Geometry: final body of the model. Coordinates: model frame, mm. Face numbers are marked on the shaded views. A direction names the side the tool comes from. Give positions to 0.01 mm unless a question says otherwise; leave off trailing zeros. Write each loop counter-clockwise with the first axis right and the second up, starting at its lowest first coordinate (ties: lowest second). Pieces come first, ordered by that corner, then holes. Notation, with made-up numbers: M 64,69.5 L 81,69.5 A17 ccw 81,94.5 Z; hole C -34.5,46.5 d7. An arc over 180 degrees is marked long. Use a Markdown table: item, result. Add a question column.
(1) Cut plane D-D (x = -25.5). Output: boundary loops of the cut face in (y, z) (3 decimals).
(2) Draft query along Y for the marked faces 3, 4 and 5. Return one class per face: released by +Y, released by -Y, zero draft, split by the parting line, or undercut.
(3) Cut plane B-B (z = 6.5). Output: boundary loops of the cut face in (x, y) (1 decimal), plus the area to 3 significant figures.
(4) Material intervals for L1, parallel to Z at x = -52.5, y = 12.7 (3 decimals); L2, parallel to Z at x = -32.5, y = 12.7; L3, parallel to X at y = 13, z = 7.25, sorted ascending.
(5) Pin query (flat end, axial travel): pin 1 Ø3 at (x, z) = (-33.5, -10) entering from +Y; pin 2 Ø2 at (y, z) = (14.5, 4.5) entering from -X; pin 3 Ø6 at (y, z) = (8, 4) entering from -X. Return the tip coordinate at first contact, or that it passes through.
(6) Reachability of the marked faces 1 and 2 from +Z, -Z, +X, -X, +Y, -Y: full face, straight path, thin tool, end or side. Return the list, or none.
(7) Cut plane A-A (y = 12.7). Output: boundary loops of the cut face in (x, z) (1 decimal), plus the area to 3 significant figures.
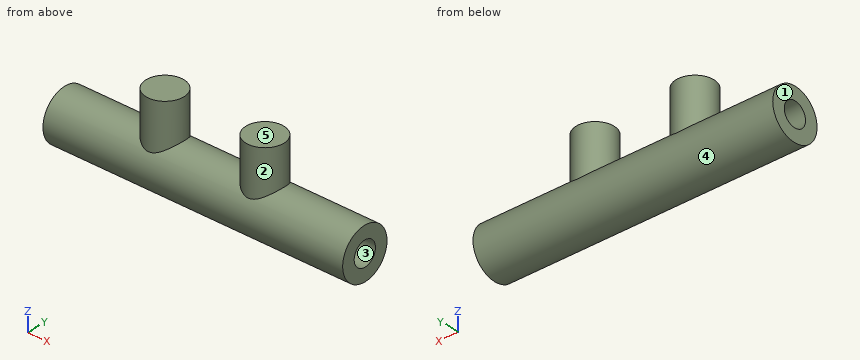
```python
from build123d import *

# Parameters (mm, degrees)
F0_R          = 6.35
F1_DEPTH      = 76.2
F2_R          = 3.048
F3_DEPTH      = 76.2
F4_R          = 4.7625
F5_DEPTH      = 9.525
F5_DEPTH_BACK = 2.54


with BuildPart() as f1:
    # F0 (on Right) → F1 (new body)
    with BuildSketch(Plane.YZ):
        with Locations((12.7, -6.664779)):
            Circle(F0_R)
    extrude(amount=-F1_DEPTH)

    # F2 (on face) → F3 (cut, through all)
    with BuildSketch(Plane.YZ):
        with Locations((12.7, -6.664779)):
            Circle(F2_R)
    extrude(amount=-F3_DEPTH, mode=Mode.SUBTRACT)

    # F4 (on Top) → F5 (join, two sides)
    with BuildSketch(Plane.XY) as f5_sk:
        with Locations((-50.8, 12.7)):
            Circle(F4_R)
        with Locations((-25.4, 12.7)):
            Circle(F4_R)
    extrude(amount=F5_DEPTH)
    extrude(f5_sk.sketch, amount=-F5_DEPTH_BACK)


solid = f1.part
```
Answer list:
| question | item | result |
|---|---|---|
| 1 | outline | M 7.939,-2.463 A6.35 ccw long 17.461,-2.463 L 17.461,9.525 L 7.939,9.525 Z; hole C 12.7,-6.665 d6.096 |
| 2 | face 3 | undercut |
| 2 | face 4 | split by the parting line |
| 2 | face 5 | zero draft |
| 3 | outline | C -50.8,12.7 d9.5; C -25.4,12.7 d9.5 |
| 3 | area | 143 mm² |
| 4 | L1 | -13.015 to -9.713, -3.617 to 9.525 |
| 4 | L2 | -13.01 to -9.71, -3.62 to -0.31 |
| 4 | L3 | -55.55 to -46.05, -30.15 to -20.65 |
| 5 | pin 1 | y = 18.78 |
| 5 | pin 2 | x = -55.49 |
| 5 | pin 3 | x = -55.25 |
| 6 | face 1 | +Z, -Z, -X, +Y, -Y |
| 6 | face 2 | +Z |
| 7 | outline | M -76.2,-13 L 0,-13 L 0,-9.7 L -76.2,-9.7 Z; M -76.2,-3.6 L 0,-3.6 L 0,-0.3 L -20.6,-0.3 L -20.6,9.5 L -30.2,9.5 L -30.2,-0.3 L -46,-0.3 L -46,9.5 L -55.6,9.5 L -55.6,-0.3 L -76.2,-0.3 Z |
| 7 | area | 691 mm² |
